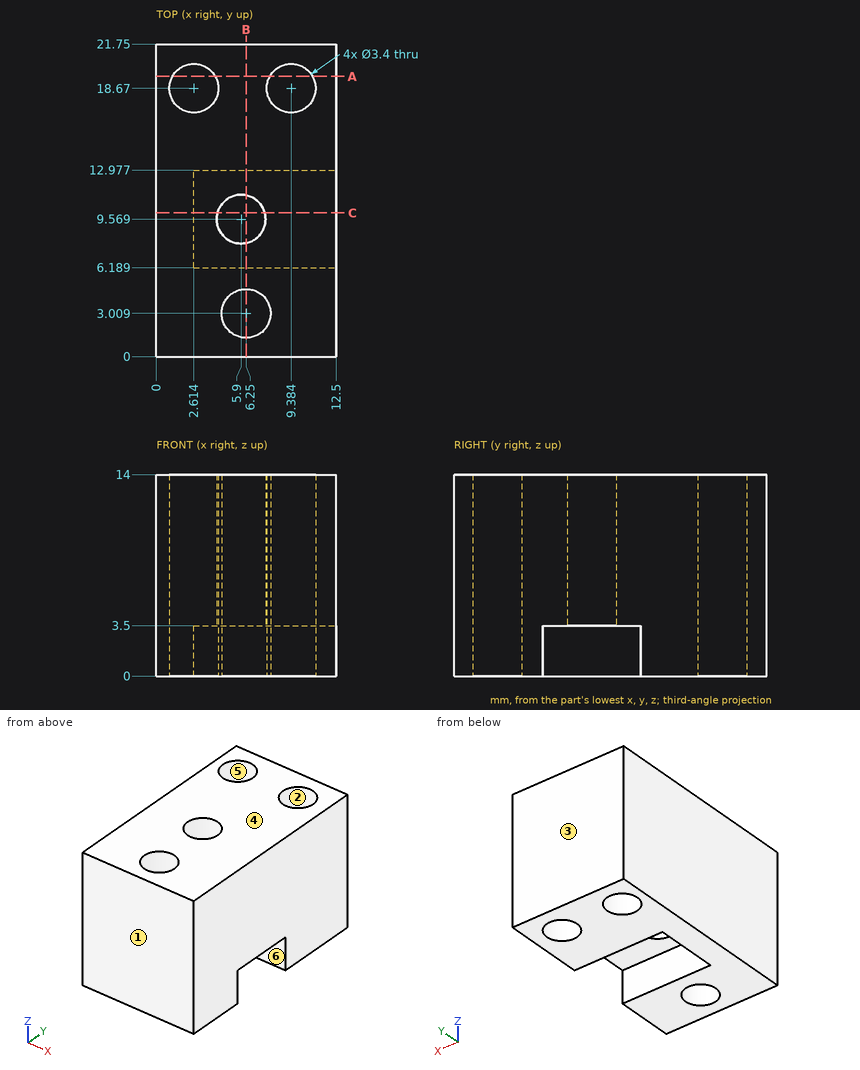
Job drawing, mm, ordinate dimensions from the low corner. One solid piece. A direction names the side the tool comes from. Give positions to 0.01 mm unless a question says otherwise; leave off trailing zeros. Order: outer loops, then holes, each group sorted by start corner. A loop starts at its lowest first (then second) coordinate and runs counter-clockwise, first axis right, second up. Notation, with made-up numbers: (29.25, 31) - (55.25, 31) arc R17 cw to (55.25, 39) - close; hole circle Ø8 at (64, 74). An arc over 180 degrees is marked (long way). Answer in a Markdown table with one row per item.
1. Saw through at B-B, the plane x = 6.25. Count the separate pieces of the cut face and the enclosed holes in it, plus the area to 3 significant figures.
Data:
| item | result |
|---|---|
| separate pieces | 3 |
| enclosed holes | 0 |
| area | 198 mm² |
2. Tool access for the marked faces 5 and 6: list every direction of +Z, -Z, +X, -X, +Y, -Y with a clear straight run to the whole face (end or side of a thin tool).
Data:
| item | result |
|---|---|
| face 5 | +Z, -Z |
| face 6 | -Z, +X |
3. Flat gauge pins, fed straight in: pin 1 (1 mm diameter, centred on y = 9.5, z = 2, fed in from +X); pin 2 (3.5 mm diameter, centred on x = 7.5, y = 8, fed in from -Z). Where does each tip first touch, or does it go through?
Data:
| item | result |
|---|---|
| pin 1 | stops at x = 2.61 |
| pin 2 | stops at z = 3.5 |
4. Saw through at C-C, the plane y = 10. Give the cut face in (x, z) (1 decimal).
Data:
| item | result |
|---|---|
| outline | (0, 0) - (2.6, 0) - (2.6, 3.5) - (4.3, 3.5) - (4.3, 14) - (0, 14) - close; (7.5, 3.5) - (12.5, 3.5) - (12.5, 14) - (7.5, 14) - close |
5. Probe probe 1 along Y at (x, z) = (6.25, 0.5); probe 2 along Z at (x, y) = (9, 6.25); probe 3 along X at (y, z) = (6.5, 3) (1 decimal). List the from-to ranges inside material, lowest first. Write a range as [from, to].
Data:
| item | result |
|---|---|
| probe 1 | y = [0, 1.31], [4.71, 6.19], [12.98, 21.75] |
| probe 2 | z = [3.5, 14] |
| probe 3 | x = [0, 2.6] |
6. Pull direction Y, two halves, no side cores. Call the marked faces 1, 2, 3 and 4: pulls with the +Y half, pulls with the -Y half, needs draft (parallel to the pull), parting line crosses it, or undercut.
Data:
| item | result |
|---|---|
| face 1 | pulls with the -Y half |
| face 2 | undercut |
| face 3 | pulls with the +Y half |
| face 4 | needs draft |
7. Saw through at A-A, the plane y = 19.5. Give the cut face in (x, z).
Data:
| item | result |
|---|---|
| outline | (0, 0) - (1.13, 0) - (1.13, 14) - (0, 14) - close; (4.1, 0) - (7.9, 0) - (7.9, 14) - (4.1, 14) - close; (10.87, 0) - (12.5, 0) - (12.5, 14) - (10.87, 14) - close |
